Geometry: see drawing. Coordinates: mm, zero at the bounding-box minimum. A direction names the side the tool comes from. Give positions to 0.01 mm unless a question says otherwise; leave off trailing zeros. Write each loop counter-clockwise with the first axis right and the second up, starting at its lowest first coordinate (ties: lowest second). Pieces come first, ordered by that corner, then holes. Notation, with made-up numbers: M 34,3.5 L 79,3.5 A13 ccw 79,22.5 Z; hole C 56.25,88.25 d10. An arc over 180 degrees is marked long. Use a Markdown table: item, result. Add a question column.
(1) Cut plane B-B (z = 14.25). Output: boundary loops of the cut face in (x, y).
(2) Cut plane C-C (y = 8.5). Output: boundary loops of the cut face in (x, z), plus the area to 3 significant figures.
(3) Pin query (flat end, axial travel): pin 1 Ø5 at (x, y) = (28, 11.5) entering from -Z; pin 2 Ø4 at (x, y) = (31, 13.5) entering from +Z; pin 3 Ø2 at (y, z) = (15.5, 11) entering from -X; pin 4 Ø5 at (y, z) = (12.5, 5.5) entering from +X. Return the tip coordinate at first contact, or that it passes through.
(4) Material intervals for L1, parallel to Z at x = 5.5, y = 23.25; L2, parallel to X at y = 14.5, z = 18.25; L3, parallel to X at y = 7.25, z = 7.25, sorted ascending.
(5) Reachability of the marked faces 4, 5 and 6 from +Z, -Z, +X, -X, +Y, -Y: full face, straight path, thin tool, end or side. Return the list, or none.
(6) Cut plane A-A (x = 12). Output: boundary loops of the cut face in (y, z).
(7) Cut plane D-D (z = 25). Output: boundary loops of the cut face in (x, y), plus the area to 3 significant figures.
(8) Draft query along Y for the marked faces 1, 2 and 3. Return one class per face: released by +Y, released by -Y, zero draft, split by the parting line, or undercut.
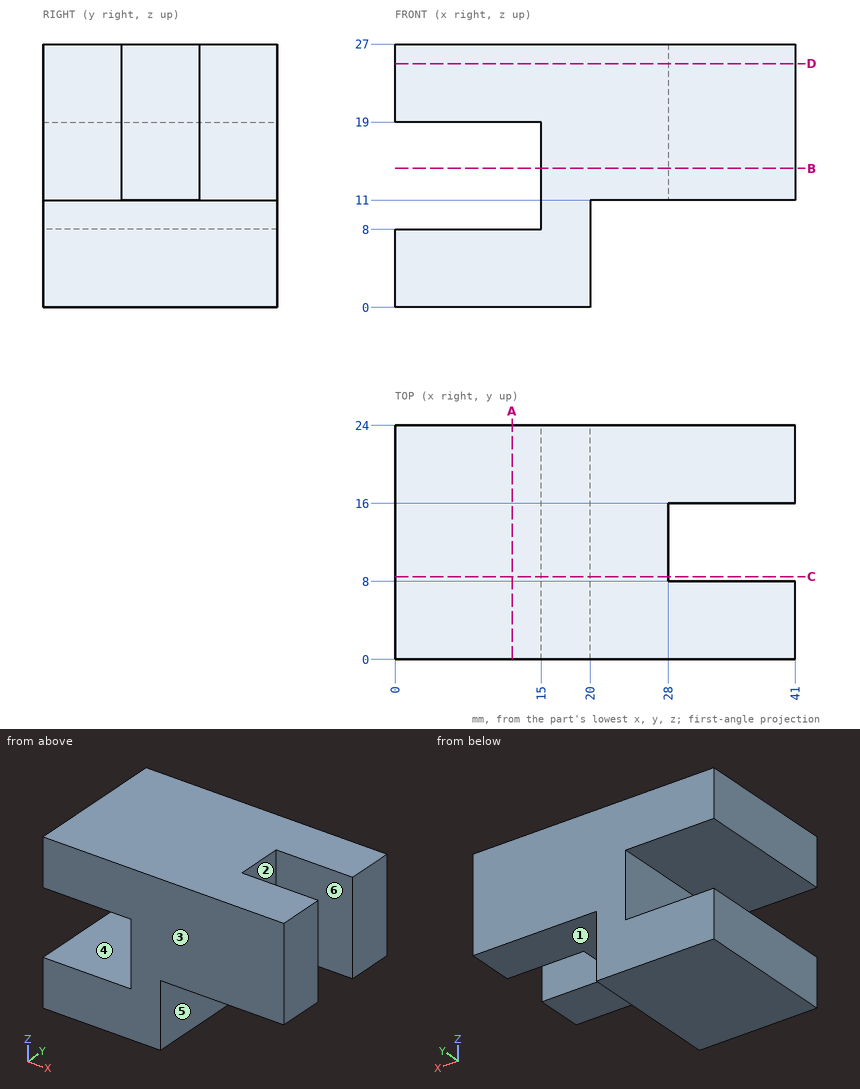
Answer list:
| question | item | result |
|---|---|---|
| 1 | outline | M 15,0 L 41,0 L 41,8 L 28,8 L 28,16 L 41,16 L 41,24 L 15,24 Z |
| 2 | outline | M 0,0 L 20,0 L 20,11 L 28,11 L 28,27 L 0,27 L 0,19 L 15,19 L 15,8 L 0,8 Z |
| 2 | area | 503 mm² |
| 3 | pin 1 | z = 11 |
| 3 | pin 2 | through |
| 3 | pin 3 | x = 15 |
| 3 | pin 4 | x = 20 |
| 4 | L1 | 0 to 8, 19 to 27 |
| 4 | L2 | 15 to 28 |
| 4 | L3 | 0 to 20 |
| 5 | face 4 | -X, +Y, -Y |
| 5 | face 5 | -Z, +X, +Y, -Y |
| 5 | face 6 | +Z, -Z, +X |
| 6 | outline | M 0,0 L 24,0 L 24,8 L 0,8 Z; M 0,19 L 24,19 L 24,27 L 0,27 Z |
| 7 | outline | M 0,0 L 41,0 L 41,8 L 28,8 L 28,16 L 41,16 L 41,24 L 0,24 Z |
| 7 | area | 880 mm² |
| 8 | face 1 | zero draft |
| 8 | face 2 | undercut |
| 8 | face 3 | released by -Y |
